Model file for the job. Use its own axes, mm. Give positions to 0.01 mm unless a question says otherwise; leave off trailing zeros. Order: outer loops, then holes, each group sorted by start corner. A loop starts at its lowest first (then second) coordinate and runs counter-clockwise, first axis right, second up. Notation, with made-up numbers: (88, 64) -> (104, 64) arc R23 cw to (104, 76) -> close; hole circle Ø1 at (39, 4.5). An arc over 180 degrees is marked (long way). Use CSV: the item, a comma, the result in double quotes. Start each with the question number.
1. Cut at A-A on x = -80. List the corners of the cut face in (y, z) (3 decimals).
2. Cut at C-C on y = 2.5. Give the number of separate pieces and of enclosed holes in the cut face, then the cut area to 3 significant figures.
3. Drop flat-ended pins along their axis: pin 1 (1 mm diameter, centred on x = -41.5, y = 1, fed in from +Z); pin 2 (1 mm diameter, centred on x = -74, y = 2.5, fed in from +Z); pin 3 (1.6 mm diameter, centred on x = -125, y = 1.5, fed in from +Z). Give the stop position or say it passes through.
4. Wall check: line 1 (X direction, y = 0.4, z = -30); line 2 (X direction, y = 0.9, z = -37); line 3 (Z direction, x = -38, y = 0.4). Give the ranges that are in metal, low to high. Write a range as from..to.
5. Cut at D-D on x = 119. List the corners of the cut face in (y, z) (1 decimal).
6. Cut at B-B on z = -101.6. List the corners of the cut face in (x, y) (1 decimal), then the cut area to 3 significant figures.
```python
from build123d import *

# Parameters (mm, degrees)
SKETCH1_R                    = 139.7
BOSS_EXTRUDE1_DEPTH          = 3.175
CUT_EXTRUDE1_DEPTH           = 198.591145108
F_3_8_0_375_DIAMETER_HOLE1_D = 9.525
CIRPATTERN2_COUNT            = 4


with BuildPart() as part:
    # Sketch1 → Boss-Extrude1 (new body)
    with BuildSketch(Plane(origin=(0, 0, 0), x_dir=(1, 0, 0), z_dir=(0, 1, 0))):
        with Locations(Location((0, 0, 0), (0, 0, 270))):
            Circle(SKETCH1_R)
    extrude(amount=BOSS_EXTRUDE1_DEPTH)

    # Sketch2 → Cut-Extrude1 (cut, through all)
    with BuildSketch(Plane(origin=(0, 3.175, 0), x_dir=(1, 0, 0), z_dir=(0, 1, 0))):
        with BuildLine():
            Line((139.618797423, 4.7625), (113.373215098, 4.7625))
            ThreePointArc((113.373215098, 4.7625), (110.319292235, 9.233847677), (105.680371094, 12.026660872))
            ThreePointArc((105.680371094, 12.026660872), (75.209645014, 75.209645014), (12.026660872, 105.680371094))
            ThreePointArc((12.026660872, 105.680371094), (9.233847677, 110.319292235), (4.7625, 113.373215098))
            Line((4.7625, 113.373215098), (4.7625, 139.618797423))
            ThreePointArc((4.7625, 139.618797423), (98.782817332, 98.782817332), (139.618797423, 4.7625))
        make_face()
        with BuildLine():
            Line((0, 88.9), (0, 0))
            Line((0, 0), (88.9, 0))
            ThreePointArc((88.9, 0), (90.866016883, 6.787606828), (96.155371094, 11.473709778))
            ThreePointArc((96.155371094, 11.473709778), (68.474452923, 68.474452923), (11.473709778, 96.155371094))
            ThreePointArc((11.473709778, 96.155371094), (6.787606828, 90.866016883), (0, 88.9))
        make_face()
    cut_extrude1 = extrude(amount=-CUT_EXTRUDE1_DEPTH, mode=Mode.SUBTRACT)

    # 3/8 (0.375) Diameter Hole1 (through all)
    with Locations(Plane(origin=(0, 3.175, 0), x_dir=(1, 0, 0), z_dir=(0, 1, 0))):
        with Locations((101.6, 0)):
            f_3_8_0_375_diameter_hole1 = Hole(F_3_8_0_375_DIAMETER_HOLE1_D / 2)

    # CirPattern2: Cut-Extrude1, 3/8 (0.375) Diameter Hole1 ×4 about axis
    cirpattern2_axis = Axis((0, 0, 0), (0, 1, 0))
    add([cut_extrude1.rotate(cirpattern2_axis, i * 360 / CIRPATTERN2_COUNT) for i in range(1, CIRPATTERN2_COUNT)], mode=Mode.SUBTRACT)
    add([f_3_8_0_375_diameter_hole1.rotate(cirpattern2_axis, i * 360 / CIRPATTERN2_COUNT) for i in range(1, CIRPATTERN2_COUNT)], mode=Mode.SUBTRACT)


solid = part.part
```
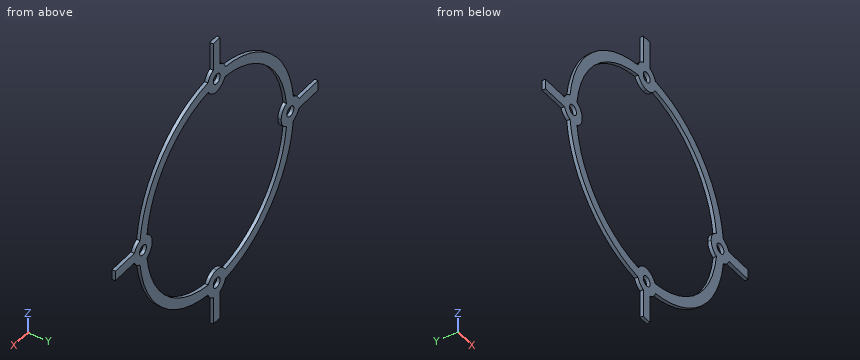
Verdict:
1,outline,"(0, -70.093) -> (3.175, -70.093) -> (3.175, -54.566) -> (0, -54.566) -> close; (0, 54.566) -> (3.175, 54.566) -> (3.175, 70.093) -> (0, 70.093) -> close"
2,separate pieces,"1"
2,enclosed holes,"5"
2,area,"7,860 mm^2"
3,pin 1,"z = 98.14"
3,pin 2,"z = 76.88"
3,pin 3,"z = 4.76"
4,line 1,"-102.04..-92.07, 92.07..102.04"
4,line 2,"-99.72..-89.49, 89.49..99.72"
4,line 3,"-99.34..-89.07, 89.07..99.34"
5,outline,"(0, -4.8) -> (3.2, -4.8) -> (3.2, 4.8) -> (0, 4.8) -> close"
6,outline,"(-31.5, 0) -> (-4.8, 0) -> (-4.8, 3.2) -> (-31.5, 3.2) -> close; (4.8, 0) -> (31.5, 0) -> (31.5, 3.2) -> (4.8, 3.2) -> close"
6,area,"170 mm^2"
